Geometry check sheet. Reference: drawing and pictorial views, mm from the part's lowest x, y, z. A direction names the side the tool comes from. Give positions to 0.01 mm unless a question says otherwise; leave off trailing zeros. Order: outer loops, then holes, each group sorted by start corner. A loop starts at its lowest first (then second) coordinate and runs counter-clockwise, first axis right, second up.
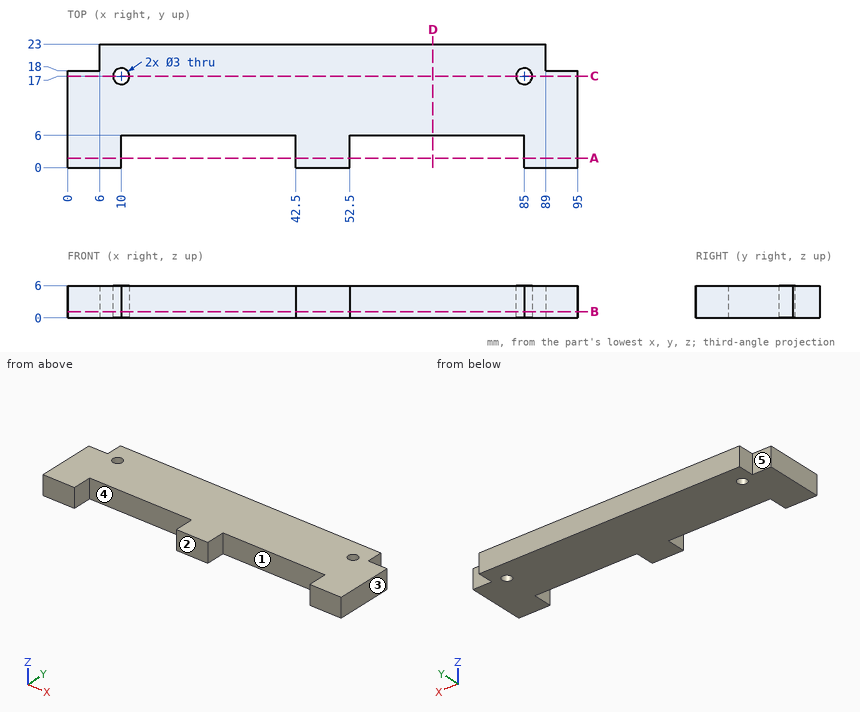
(1) Cross-section at A-A on y = 1.75. Enter the section's corners in (x, z), then the cut area to 3 significant figures.
Response values:
outline: (0, 0) - (10, 0) - (10, 6) - (0, 6) - close; (42.5, 0) - (52.5, 0) - (52.5, 6) - (42.5, 6) - close; (85, 0) - (95, 0) - (95, 6) - (85, 6) - close
area: 180 mm2
(2) Set-up check for the marked faces 1 and 2: record each of +Z, -Z, +X, -X, +Y, -Y from which the full face is reachable in a straight line by a thin tool's end or side.
Response values:
face 1: +Z, -Z, -Y
face 2: +Z, -Z, +X, -X, -Y
(3) Gauge pin test, flat ends, axial feed: pin 1 Ø3 at (y, z) = (1.5, 3.5) entering from -X; pin 2 Ø1.8 at (x, z) = (31, 4.5) entering from -Y; pin 3 Ø3 at (x, z) = (91.5, 3.5) entering from +Y. Record the tip position at first contact, or that the pin passes through.
Response values:
pin 1: stops at x = 0
pin 2: stops at y = 6
pin 3: stops at y = 18
(4) Release check for a two-part mould opening along X. For the marked faces 3, 4 and 5 record: released by +X, released by -X, zero draft, split by the parting line, or undercut.
Response values:
face 3: released by +X
face 4: undercut
face 5: zero draft
(5) Cross-section at C-C on y = 17. Enter the section's corners in (x, z), then the cut area to 3 significant figures.
Response values:
outline: (0, 0) - (8.5, 0) - (8.5, 6) - (0, 6) - close; (11.5, 0) - (83.5, 0) - (83.5, 6) - (11.5, 6) - close; (86.5, 0) - (95, 0) - (95, 6) - (86.5, 6) - close
area: 534 mm2
(6) Cross-section at D-D on x = 68. Enter the section's corners in (y, z), then the cut area to 3 significant figures.
Response values:
outline: (6, 0) - (23, 0) - (23, 6) - (6, 6) - close
area: 102 mm2
(7) Cross-section at B-B on z = 1.15. Enter the section's corners in (x, y).
Response values:
outline: (0, 0) - (10, 0) - (10, 6) - (42.5, 6) - (42.5, 0) - (52.5, 0) - (52.5, 6) - (85, 6) - (85, 0) - (95, 0) - (95, 18) - (89, 18) - (89, 23) - (6, 23) - (6, 18) - (0, 18) - close; hole circle Ø3 at (10, 17); hole circle Ø3 at (85, 17)
(8) Material ranges on L1, parallel to X at y = 5.25, z = 3.65; L2, parallel to X at y = 16.5, z = 5.1; L3, parallel to Y at x = 65.5, z = 2.95, recorded low to high.
Response values:
L1: x = 0 to 10, 42.5 to 52.5, 85 to 95
L2: x = 0 to 8.59, 11.41 to 83.59, 86.41 to 95
L3: y = 6 to 23
